Input: part model. Units: mm. Frame: model coordinates. A direction names the side the tool comes from. Coordinates: 2 decimals unless noted, no trailing zeros. Order: outer loops, then holes, each group sorted by start corner. A loop starts at its lowest first (then second) coordinate and runs counter-clockwise, first axis right, second up. Notation, with made-up numbers: (-20.75, 85.5) -> (-13.75, 85.5) arc R29 cw to (-13.75, 119.5) -> close; hole circle Ø1 at (87.5, 50.25). An arc over 180 degrees is marked (long way). Use one line per item in the form item = value. Start each with the question number.
1) Section query D-D on z = 0.7. Count the separate pieces of the cut face and the enclosed holes in it, then the cut area to 3 significant figures.
2) Pin query (flat end, axial travel): pin 1 (5 mm diameter, centred on x = 75.692, y = 0, fed in from +Z). Return the tip coordinate at first contact, or that it passes through.
3) Section query B-B on x = 36.5. Output: boundary loops of the cut face in (y, z), then the cut area to 3 significant figures.
4) Draft query along X for faces 1 (the flat face through (-67, 19, 0)), 2 (the cylindrical face through (58.318, 57.705, 0.493)), 3 (the flat face through (70.324, 27.755, 0.507)). Return one class per face: pulls with the +X half, pulls with the -X half, needs draft (parallel to the pull), parting line crosses it, or undercut.
5) Access query for faces 4 (the flat face through (69.52, 30.17, 0.51)), 5 (the cylindrical face through (-58.318, -57.705, 0.493)). Directions: +Z, -Z, +X, -X, +Y, -Y. A direction counts if a zero-diameter tool reaches every point of the face in a straight line with its end or side. Return the directions, or none.
6) Ray query, line 1 along Y through (x, z) = (-1, 0.8); line 2 along Y through (x, z) = (54.5, 0.6); line 3 along X through (y, z) = (-53, 0.8) (3 decimals). Return the intervals inside material, ascending.
7) Section query C-C on y = 64. Output: boundary loops of the cut face in (x, z).
8) Section query A-A on x = 0. Output: boundary loops of the cut face in (y, z).
from build123d import *

# Parameters (mm, degrees)
SKETCH4_R           = 82.042
BOSS_EXTRUDE2_DEPTH = 1
SKETCH5_R           = 69.342
CUT_EXTRUDE5_DEPTH  = 2
SKETCH6_R           = 3.175
CUT_EXTRUDE6_DEPTH  = 2
CIRPATTERN1_COUNT   = 8
CUT_EXTRUDE11_DEPTH = 2


with BuildPart() as part:
    # Sketch4 → Boss-Extrude2 (new body)
    with BuildSketch(Plane.XY):
        Circle(SKETCH4_R)
    extrude(amount=BOSS_EXTRUDE2_DEPTH)

    # Sketch5 → Cut-Extrude5 (cut, through all)
    with BuildSketch(Plane.XY.offset(1)):
        Circle(SKETCH5_R)
    extrude(amount=-CUT_EXTRUDE5_DEPTH, mode=Mode.SUBTRACT)

    # Sketch6 → Cut-Extrude6 (cut, through all)
    with BuildSketch(Plane.XY.offset(1)):
        with Locations((75.692, 0)):
            Circle(SKETCH6_R)
    cut_extrude6 = extrude(amount=-CUT_EXTRUDE6_DEPTH, mode=Mode.SUBTRACT)

    # CirPattern1: Cut-Extrude6 ×8 about axis
    cirpattern1_axis = Axis((0, 0, 0), (0, 0, 1))
    for i in range(1, CIRPATTERN1_COUNT):
        add(cut_extrude6.rotate(cirpattern1_axis, i * 360 / CIRPATTERN1_COUNT), mode=Mode.SUBTRACT)

    # Sketch8 → Cut-Extrude11 (cut, through all)
    with BuildSketch(Plane.XY.offset(1)):
        Polygon((78.830897666, 34.027465042), (60.057665565, 26.251337696), (61.029681484, 23.904683683), (79.802913584, 31.680811029), align=None)
        Polygon((32.812445144, 75.89758015), (30.465791131, 76.869596069), (29.979783172, 75.696269062), (32.326437185, 74.724253144), align=None)
        Polygon((-30.465791131, 76.869596069), (-32.812445144, 75.89758015), (-32.326437185, 74.724253144), (-29.979783172, 75.696269062), align=None)
        Polygon((-75.89758015, 32.812445144), (-76.869596069, 30.465791131), (-75.696269062, 29.979783172), (-74.724253144, 32.326437185), align=None)
        Polygon((-76.869596069, -30.465791131), (-75.89758015, -32.812445144), (-74.724253144, -32.326437185), (-75.696269062, -29.979783172), align=None)
        Polygon((-32.812445144, -75.89758015), (-30.465791131, -76.869596069), (-29.979783172, -75.696269062), (-32.326437185, -74.724253144), align=None)
        Polygon((30.465791131, -76.869596069), (32.812445144, -75.89758015), (32.326437185, -74.724253144), (29.979783172, -75.696269062), align=None)
        Polygon((75.89758015, -32.812445144), (76.869596069, -30.465791131), (75.696269062, -29.979783172), (74.724253144, -32.326437185), align=None)
    extrude(amount=-CUT_EXTRUDE11_DEPTH, mode=Mode.SUBTRACT)


solid = part.part
Answers below:
q1.separate_pieces = 1
q1.enclosed_holes = 8
q1.area = 5,740 mm^2
q2.pin_1 = through
q3.outline = (-73.48, 0) -> (-58.96, 0) -> (-58.96, 1) -> (-73.48, 1) -> close; (58.96, 0) -> (73.48, 0) -> (73.48, 1) -> (58.96, 1) -> close
q3.area = 29.0 mm^2
q4.face_1 = needs draft
q4.face_2 = pulls with the +X half
q4.face_3 = undercut
q5.face_4 = +Z, -Z
q5.face_5 = +Z, -Z, -X, -Y
q6.line_1 = -82.04 to -78.71, -72.68 to -69.33, 69.33 to 72.68, 78.71 to 82.04
q6.line_2 = -61.32 to -56.54, -50.5 to -42.87, 42.87 to 50.5, 56.54 to 61.32
q6.line_3 = -62.625 to -56.654, -50.391 to -44.714, 44.714 to 50.391, 56.654 to 62.625
q7.outline = (-51.33, 0) -> (-26.69, 0) -> (-26.69, 1) -> (-51.33, 1) -> close; (26.69, 0) -> (51.33, 0) -> (51.33, 1) -> (26.69, 1) -> close
q8.outline = (-82.04, 0) -> (-78.87, 0) -> (-78.87, 1) -> (-82.04, 1) -> close; (-72.52, 0) -> (-69.34, 0) -> (-69.34, 1) -> (-72.52, 1) -> close; (69.34, 0) -> (72.52, 0) -> (72.52, 1) -> (69.34, 1) -> close; (78.87, 0) -> (82.04, 0) -> (82.04, 1) -> (78.87, 1) -> close
